Can you work these out from the model? Positions are in its coordinate system, mm. A direction names the side the tool comes from. Coordinates: 2 decimals unless noted, no trailing zeros. Write each loop counter-clockwise with the first axis right and the second up, starting at its lowest first coordinate (ties: lowest second). Pieces come first, ordered by that corner, then holes. Notation, with made-up numbers: (-32.75, -14) - (-12.75, -14) arc R34 ccw to (-12.75, 23) - close; hole circle Ø6 at (6.5, 81). An arc over 180 degrees is marked (long way). Use one line per item in the form item = value. Start each with the question number.
(1) Thinking about a two-plate mould opening in X: for faces 4 (the face through (475.1, 758.58, -250.44)), 5 (the face through (0, 201, -388)), 6 (the face through (764, 556, -508)), which applies, pulls with the +X half, pulls with the -X half, needs draft (parallel to the pull), parting line crosses it, or undercut?
(2) For pin 1 Ø2 at (x, y) = (1121, 368.5) entering from -Z; pin 2 Ø8 at (x, z) = (1245, -744) entering from +Y; pin 3 Ø1.5 at (x, z) = (782, -169.5) entering from +Y, each with a flat end and sliding along its axis, tell me the tip position at first contact or that it passes through.
(3) If we section it at B-B on z = -305.5: Please give me the cut outline in (x, y), then the cut area to 3 significant figures.
(4) If I drill on probe 1 along Y at (x, z) = (508, -251); probe 2 along Z at (x, y) = (223, 883); probe 3 along X at (y, z) = (472.5, -190.5), over which ranges is the centre line in solid material (lowest first)? Write a range as from..to.
(5) On a 3-axis mill with a long thin cutter (end or side, diameter ignored), from which of +Z, -Z, +X, -X, +Y, -Y can I reach the whole of each face in a straight line? I mean faces 1 (the face through (1158, 508, -250)), 2 (the face through (764, 0, -501)), 3 (the face through (764, 254, -758)). Say none if no direction works.
(6) If we section it at A-A on x = 508: Please give me the cut outline in (y, z), then the cut area to 3 significant figures.
(7) If we section it at C-C on y = 560.5: Please give me the cut outline in (x, z).
(8) If we section it at D-D on z = -550.5: Please give me the cut outline in (x, y).
```python
from build123d import *

# Parameters (mm, degrees)
SKETCH1_W           = 1016
SKETCH1_H           = 254
BOSS_EXTRUDE1_DEPTH = 1549.4
SKETCH2_R           = 252.73
BOSS_EXTRUDE2_DEPTH = 508


with BuildPart() as part:
    # Sketch1 → Boss-Extrude1 (new body)
    with BuildSketch(Plane(origin=(0, 0, 0), x_dir=(0, 0, -1), z_dir=(1, 0, 0))):
        with Locations((508, 127)):
            Rectangle(SKETCH1_W, SKETCH1_H)
    extrude(amount=BOSS_EXTRUDE1_DEPTH)

    # Sketch2 → Boss-Extrude2 (add)
    with BuildSketch(Plane.XY):
        with BuildLine():
            Line((0, 508), (0, 254))
            Line((0, 254), (1549.4, 254))
            ThreePointArc((1549.4, 254), (1475.005122421, 433.605122421), (1295.4, 508))
            Line((1295.4, 508), (1016, 508))
            ThreePointArc((1016, 508), (508, 1016), (0, 508))
        make_face()
        with Locations((508, 508)):
            Circle(SKETCH2_R, mode=Mode.SUBTRACT)
    extrude(amount=-BOSS_EXTRUDE2_DEPTH)


solid = part.part
```
Reported:
q1.face_4 = undercut
q1.face_5 = pulls with the -X half
q1.face_6 = needs draft
q2.pin_1 = -508
q2.pin_2 = 254
q2.pin_3 = 936.25
q3.outline = (0, 0) - (1549.4, 0) - (1549.4, 254) arc R254 ccw to (1295.4, 508) - (1016, 508) arc R508 ccw to (0, 508) - close; hole circle Ø505.46 at (508, 508)
q3.area = 978,000 mm2
q4.probe_1 = 0..255.27, 760.73..1016
q4.probe_2 = -508..0
q4.probe_3 = 0..257.78, 758.22..1424.91
q5.face_1 = +Z, -Z, +X, +Y
q5.face_2 = +Z, -Z, +X, -X, -Y
q5.face_3 = -Z, +X, -X, +Y
q6.outline = (0, -1016) - (254, -1016) - (254, -508) - (255.27, -508) - (255.27, 0) - (0, 0) - close; (760.73, -508) - (1016, -508) - (1016, 0) - (760.73, 0) - close
q6.area = 388,000 mm2
q7.outline = (2.72, -508) - (260.78, -508) - (260.78, 0) - (2.72, 0) - close; (755.22, -508) - (1013.28, -508) - (1013.28, 0) - (755.22, 0) - close
q8.outline = (0, 0) - (1549.4, 0) - (1549.4, 254) - (0, 254) - close
